For this review, use the dimensioned drawing (mm, ordinates from the lowest corner) and the shaded views. A direction names the side the tool comes from. Round coordinates to 2 decimals unless told otherwise and drop trailing zeros. Write each loop counter-clockwise with the first axis right and the second up, starting at its lowest first coordinate (ties: lowest second). Pieces come first, ordered by that corner, then holes.
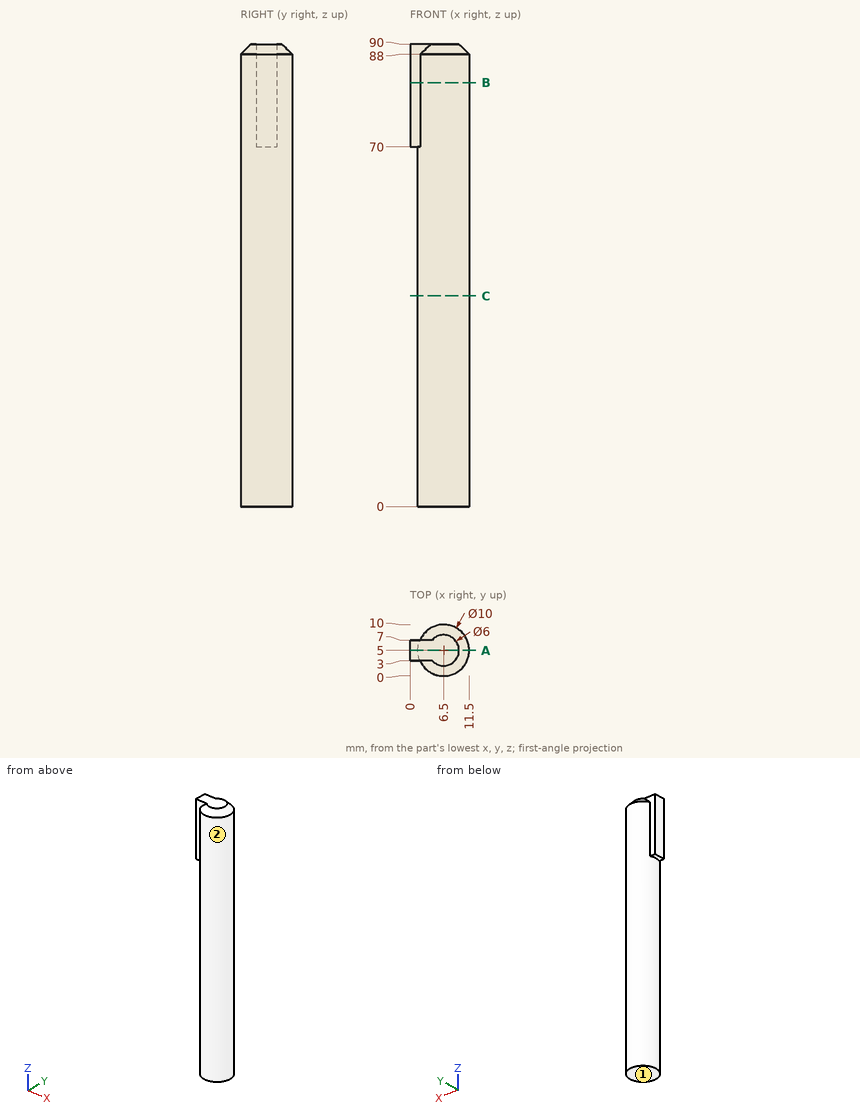
(1) We need section C-C, the plane z = 41. Give the boundary of the cut face in (x, y), and give its area (3 significant figures).
Geometry check:
outline: circle Ø10 at (6.5, 5)
area: 78.5 mm2
(2) We need section A-A, the plane y = 5. Give the boundary of the cut face in (x, z), and give its area (3 significant figures).
Geometry check:
outline: (0, 70) - (1.5, 70) - (1.5, 0) - (11.5, 0) - (11.5, 88) - (9.5, 90) - (0, 90) - close
area: 928 mm2
(3) For the marked faces 1 and 2, list the 3-axis set-ups (+Z, -Z, +X, -X, +Y, -Y) from which the entire face can be reached by the end or side of a thin tool; tool diameter is ignored.
Geometry check:
face 1: -Z, +X, -X, +Y, -Y
face 2: -Z
(4) For pin 1 Ø4.5 at (x, z) = (1.5, 80) entering from -Y; pin 2 Ø1 at (x, z) = (4.5, 67) entering from -Y; pin 3 Ø3 at (y, z) = (6.5, 34.5) entering from -X, all flat-tipped, find the tip position at first contact; note any pin that passes through.
Geometry check:
pin 1: stops at y = 0.82
pin 2: stops at y = 0.23
pin 3: stops at x = 1.5
(5) We need section B-B, the plane z = 82.5. Give the boundary of the cut face in (x, y).
Geometry check:
outline: (0, 3) - (1.92, 3) arc R5 ccw (long way) to (1.92, 7) - (0, 7) - close
(6) For line 1 along X through (y, z) = (5.25, 5.5); line 2 along Z through (x, y) = (0.5, 4.5); line 3 along Y through (x, z) = (5.5, 29.5), list the stretches that pass through material, from the lowest coordinate up.
Geometry check:
line 1: x = 1.51 to 11.49
line 2: z = 70 to 90
line 3: y = 0.1 to 9.9
